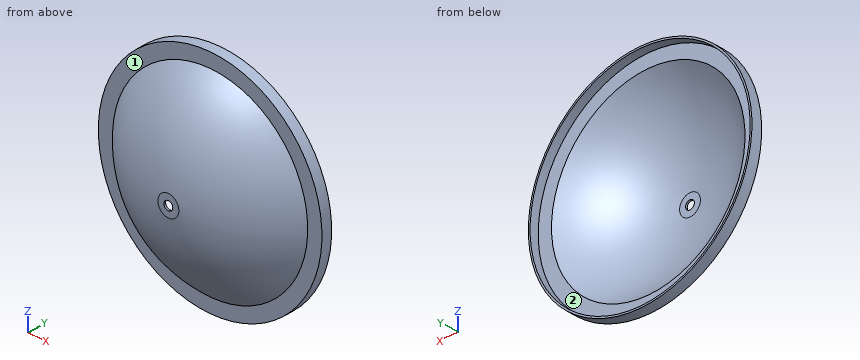
from build123d import *


with BuildPart() as part:
    # Sketch1 → Revolve2 (revolve)
    with BuildSketch(Plane.XY, mode=Mode.PRIVATE) as revolve2_sk:
        with BuildLine():
            Line((-2.5, -72.753006811), (-6, -72.753006811))
            ThreePointArc((-6, -72.753006811), (-33.50186891, -64.858498129), (-55.856960175, -47))
            Line((-55.856960175, -47), (-64, -47))
            Line((-64, -47), (-64, -41))
            Line((-64, -41), (-63, -41))
            Line((-63, -41), (-63, -46))
            Line((-63, -46), (-55.389529697, -46))
            ThreePointArc((-55.389529697, -46), (-33.267182398, -63.853696646), (-5.958692274, -71.753006811))
            Line((-5.958692274, -71.753006811), (-2.5, -71.753006811))
            Line((-2.5, -71.753006811), (-2.5, -72.753006811))
        make_face()
    revolve(revolve2_sk.sketch.rotate(Axis((0, 36.298912202, 0), (0, -1, 0)), 270), axis=Axis((0, 36.298912202, 0), (0, -1, 0)))


solid = part.part
Geometry: final body of the model. Coordinates: model frame, mm. Face numbers are marked on the shaded views. Round coordinates to 2 decimals unless told otherwise and drop trailing zeros. Loops run counter-clockwise (first coordinate to the right, second up) from the corner with the lowest first, then second, coordinate; pieces in that order, holes last. Notation, with made-up numbers: (8, 63) - (60, 63) arc R28 cw to (60, 84) - close; hole circle Ø6 at (33.5, -37.5). An arc over 180 degrees is marked (long way). Write each question's results on one line, items separated by ' | '. Start each with the question number.
1) Cut plane A-A on x = 0. Return loops of the section in (y, z).
2) Mould query, pull axis Z, two halves, no side actions, for the marked faces 1 and 2. Classes: released by +Z, released by -Z, zero draft, split by the parting line, or undercut.
3) Cut plane D-D on y = -52. Return loops of the section in (x, z).
4) Cut plane C-C on z = 13. Return loops of the section in (x, y), then the cut area to 3 significant figures.
5) First-contact query: P1, Ø13, axis at x = -1.5, z = 1.5, coming from the +Y side; P2, Ø1, axis at y = -58, z = 22, coming from the +X side; P3, Ø4, axis at x = -23, z = 24.5, coming from the -Y side. Flat tips, straight axial feed; report the tip coordinate or a pass-through.
6) Cut plane B-B on z = 0. Return loops of the section in (x, y), then the cut area to 3 significant figures.
7) Line query: probe 1 along X at (y, z) = (-44.3, 0); probe 2 along X at (y, z) = (-60, 1.5); probe 3 along Z at (x, y) = (1, -65.5). Output: solid intervals per line, ascending. Write a range as [from, to].
Verdict:
1) outline: (-72.75, -6) arc R73 ccw to (-47, -55.86) - (-47, -64) - (-41, -64) - (-41, -63) - (-46, -63) - (-46, -55.39) arc R72 cw to (-71.75, -5.96) - (-71.75, -2.5) - (-72.75, -2.5) - close; (-72.75, 2.5) - (-71.75, 2.5) - (-71.75, 5.96) arc R72 cw to (-46, 55.39) - (-46, 63) - (-41, 63) - (-41, 64) - (-47, 64) - (-47, 55.86) arc R73 ccw to (-72.75, 6) - close
2) face 1: zero draft | face 2: undercut
3) outline: circle Ø102.47 at (0, 0); hole circle Ø99.6 at (0, 0)
4) outline: (-62.67, -47) - (-54.32, -47) arc R71.83 ccw to (54.32, -47) - (62.67, -47) - (62.67, -41) - (61.64, -41) - (61.64, -46) - (53.84, -46) arc R70.82 cw to (-53.84, -46) - (-61.64, -46) - (-61.64, -41) - (-62.67, -41) - close | area: 152 mm2
5) P1: stops at y = -71.48 | P2: stops at x = 39.28 | P3: stops at y = -65.8
6) outline: (-64, -47) - (-55.86, -47) arc R73 ccw to (-6, -72.75) - (-2.5, -72.75) - (-2.5, -71.75) - (-5.96, -71.75) arc R72 cw to (-55.39, -46) - (-63, -46) - (-63, -41) - (-64, -41) - close; (2.5, -72.75) - (6, -72.75) arc R73 ccw to (55.86, -47) - (64, -47) - (64, -41) - (63, -41) - (63, -46) - (55.39, -46) arc R72 cw to (5.96, -71.75) - (2.5, -71.75) - close | area: 149 mm2
7) probe 1: x = [-64, -63], [63, 64] | probe 2: x = [-41.55, -39.77], [39.77, 41.55] | probe 3: z = [-32.21, -29.88], [29.88, 32.21]
